Source: CAD feature listing. Evaluate the final solid. Frame: model axes, mm. Face numbers are marked on the shaded views. A direction names the side the tool comes from. Give positions to 0.01 mm unless a question says otherwise; leave off trailing zeros. Order: outer loops, then holes, each group sorted by start corner. A loop starts at its lowest first (then second) coordinate and runs counter-clockwise, first axis right, second up.
1) Section A-A, the plane x = 10. Return loops of the section in (y, z), plus the area to 4 significant figures.
2) Section C-C, the plane z = 1.45. Return loops of the section in (x, y), plus the area to 3 significant figures.
3) Material intervals for line 1 (Y direction, x = 16, z = 4.05); line 2 (Y direction, x = 10, z = 2.05), sorted ascending.
4) Draft query along X for the marked faces 3, 4 and 5. Return one class per face: released by +X, released by -X, zero draft, split by the parting line, or undercut.
5) Section B-B, the plane y = 6. Return loops of the section in (x, z), plus the area to 3 significant figures.
6) Access query for the marked faces 1 and 2. Directions: +Z, -Z, +X, -X, +Y, -Y. A direction counts if a zero-diameter tool reaches every point of the face in a straight line with its end or side. Return the directions, or none.
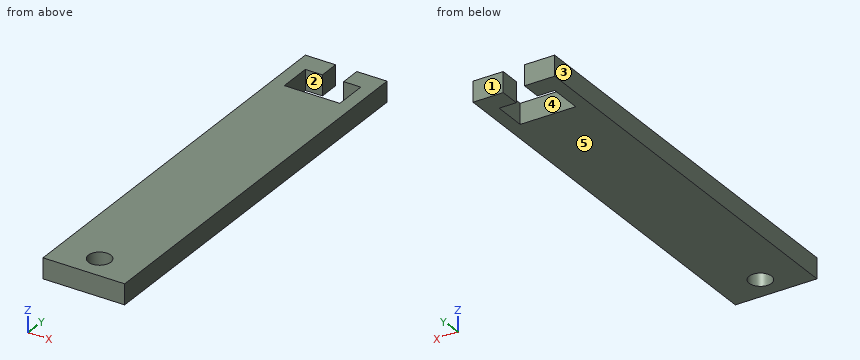
Autodesk Inventor part; units mm, degrees
ref_plane "YZ Plane" through (0, 0, 0) normal (1, 0, 0) x (0, 1, 0)
ref_plane "XZ Plane" through (0, 0, 0) normal (0, 1, 0) x (-1, 0, 0)
ref_plane "XY Plane" through (0, 0, 0) normal (0, 0, 1) x (1, 0, 0)
sketch "Sketch1" plane through (0, 0, 0) normal (0, 0, 1) x (1, 0, 0)
  line L0 (0, 0) -> (20, 0)
  line L1 (20, 0) -> (20, 100)
  line L2 (20, 100) -> (0, 100)
  line L3 (0, 100) -> (0, 0)
  dimension "d0" = 20
  dimension "d1" = 100
extrude "Extrusion1" add sketch "Sketch1" along normal blind 5
sketch "Sketch2" plane through (0, 0, 5) normal (0, 0, 1) x (1, 0, 0)
  line L0 (20, 100) -> (0, 100)
  line L1 (7.4, 100) -> (7.4, 95)
  line L2 (7.4, 95) -> (3.2, 95)
  line L3 (3.2, 95) -> (3.2, 87)
  line L4 (3.2, 87) -> (10, 87)
  line L5 (10, 87) -> (10, 204.0933)
  line L6 (7.4, 100) -> (10, 100)
  line L7 (20, 0) -> (20, 100)
  line L8 (0, 100) -> (20, 100)
  line L9 (12.6, 100) -> (12.6, 95)
  line L10 (12.6, 95) -> (16.8, 95)
  line L11 (16.8, 95) -> (16.8, 87)
  line L12 (16.8, 87) -> (10, 87)
  line L13 (12.6, 100) -> (10, 100)
  circle A0 centre (10, 6) radius 2.75
  line L14 (0, 0) -> (20, 0)
  dimension "d4" = 2.6
  dimension "d5" = 8
  dimension "d6" = 5
  dimension "d7" = 10
  dimension "d8" = 4.2
  dimension "d11" = 5.5
  dimension "d12" = 10
  dimension "d13" = 6
extrude "Extrusion2" cut sketch "Sketch2" against normal blind 5
properties part number "Leg1" material "Wood (Birch)"
From the geometry:
1. outline: (0, 0) - (3.25, 0) - (3.25, 5) - (0, 5) - close; (8.75, 0) - (87, 0) - (87, 5) - (8.75, 5) - close
1. area: 407.5 mm2
2. outline: (0, 0) - (20, 0) - (20, 100) - (12.6, 100) - (12.6, 95) - (16.8, 95) - (16.8, 87) - (3.2, 87) - (3.2, 95) - (7.4, 95) - (7.4, 100) - (0, 100) - close; hole circle Ø5.5 at (10, 6)
2. area: 1,840 mm2
3. line 1: y = 0 to 87, 95 to 100
3. line 2: y = 0 to 3.25, 8.75 to 87
4. face 3: released by -X
4. face 4: undercut
4. face 5: zero draft
5. outline: (0, 0) - (7.25, 0) - (7.25, 5) - (0, 5) - close; (12.75, 0) - (20, 0) - (20, 5) - (12.75, 5) - close
5. area: 72.5 mm2
6. face 1: +Z, -Z, +X, -X, +Y
6. face 2: +Z, -Z
